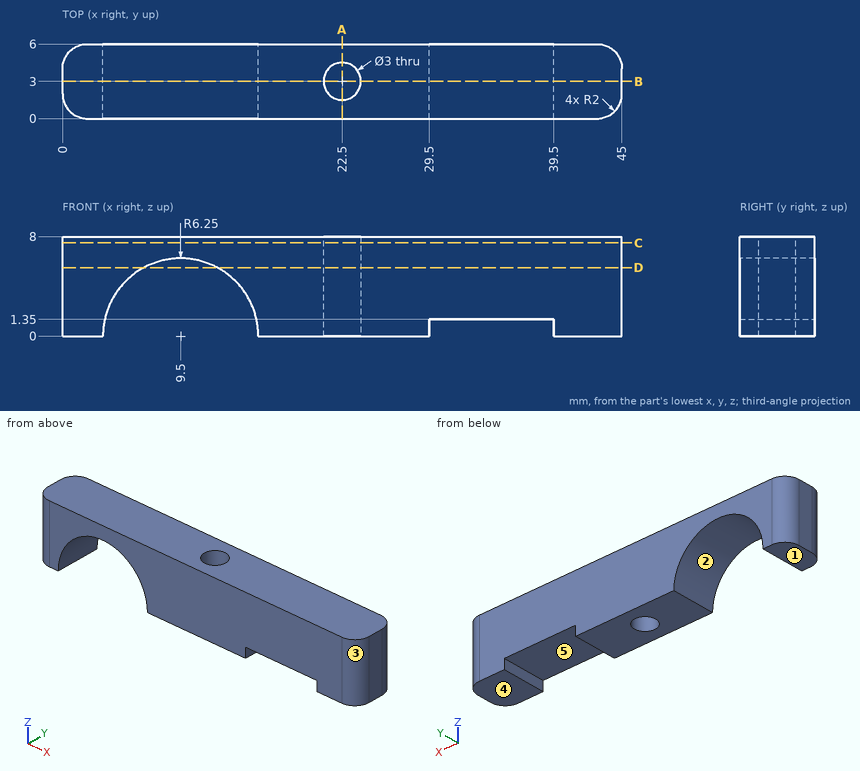
Drawing for the job (mm, zero at the part's lowest x, y, z). A direction names the side the tool comes from. Give positions to 0.01 mm unless a question says otherwise; leave off trailing zeros. Loops run counter-clockwise (first coordinate to the right, second up) from the corner with the lowest first, then second, coordinate; pieces in that order, holes last. Notation, with made-up numbers: M -34.75,89.5 L 16.25,89.5 A24 cw 16.25,108.5 Z; hole C -10,34 d2. An arc over 180 degrees is marked long. Use one line per item in the form item = value.
Item 1: Flat gauge pins, fed straight in: pin 1 (2 mm diameter, centred on x = 13.5, y = 1.5, fed in from -Z); pin 2 (1.1 mm diameter, centred on y = 3.5, z = 0.5, fed in from -X). Where does each tip first touch, or does it go through?
Determined:
pin_1 = 3.75
pin_2 = 0
Item 2: Which spindle directions (+Z, -Z, +X, -X, +Y, -Y) get a long thin tool onto all of the face, cutting with end or side? Do the marked faces 4 and 5. Say none if no direction does.
Determined:
face_4 = -Z, +X, -X, +Y, -Y
face_5 = -Z, +Y, -Y
Item 3: Slice it at A-A (x = 22.5). List the corners of the cut face in (y, z), plus the area to 3 significant figures.
Determined:
outline = M 0,0 L 1.5,0 L 1.5,8 L 0,8 Z; M 4.5,0 L 6,0 L 6,8 L 4.5,8 Z
area = 24.0 mm2
Item 4: Slice it at B-B (y = 3). List the corners of the cut face in (x, z).
Determined:
outline = M 0,0 L 3.25,0 A6.25 cw 15.75,0 L 21,0 L 21,8 L 0,8 Z; M 24,0 L 29.5,0 L 29.5,1.35 L 39.5,1.35 L 39.5,0 L 45,0 L 45,8 L 24,8 Z
Item 5: Two-plate mould, pull along X, no slides. Class the marked faces 1, 2 and 3: pulls with the +X half, pulls with the -X half, needs draft (parallel to the pull), parting line crosses it, or undercut.
Determined:
face_1 = needs draft
face_2 = undercut
face_3 = pulls with the +X half
Item 6: Slice it at D-D (z = 5.5). List the corners of the cut face in (x, y).
Determined:
outline = M 0,2 A2 ccw 2,0 L 6.53,0 L 6.53,6 L 2,6 A2 ccw 0,4 Z; M 12.47,0 L 43,0 A2 ccw 45,2 L 45,4 A2 ccw 43,6 L 12.47,6 Z; hole C 22.5,3 d3
Item 7: Drill centre lines: probe 1 along Y at (x, z) = (22.5, 4); probe 2 along X at (y, z) = (3.25, 2.25); probe 3 along X at (y, z) = (2, 2.25). Where is each one in solid material? Low to high. Write a range as from..to.
Determined:
probe_1 = 0..1.5, 4.5..6
probe_2 = 0..3.67, 15.33..21.02, 23.98..45
probe_3 = 0..3.67, 15.33..21.38, 23.62..45
Item 8: Slice it at C-C (z = 7.5). List the corners of the cut face in (x, y).
Determined:
outline = M 0,2 A2 ccw 2,0 L 43,0 A2 ccw 45,2 L 45,4 A2 ccw 43,6 L 2,6 A2 ccw 0,4 Z; hole C 22.5,3 d3
